Work out the finished part from the listing and answer in its coordinate system (mm). A direction names the side the tool comes from. Round coordinates to 2 decimals unless told otherwise and drop trailing zeros. Loops run counter-clockwise (first coordinate to the right, second up) from the corner with the lowest first, then second, coordinate; pieces in that order, holes last. Notation, with made-up numbers: (-29.75, -15) - (13.25, -15) arc R13 cw to (13.25, -3) - close; hole circle Ø7 at (17, 37.25). An arc over 180 degrees is marked (long way). Return JSON: item names as keys, results as strings.
from build123d import *

# Parameters (mm, degrees)
SKETCH1_R                         = 24.765
BOSS_EXTRUDE1_DEPTH               = 19.05
SKETCH2_OUTSIDE_W                 = 66.048
SKETCH2_OUTSIDE_H                 = 66.048
CUT_EXTRUDE1_DEPTH                = 9.525
F_1_4_20_TAPPED_HOLE5_D           = 5.1054
F_1_4_20_TAPPED_HOLE5_DEPTH       = 7.62
F_1_4_20_TAPPED_HOLE5_CSINK_D     = 6.731
F_1_4_20_TAPPED_HOLE5_CSINK_ANGLE = 90
F_1_4_20_TAPPED_HOLE5_TIP         = 1.533816902


with BuildPart() as part:
    # Sketch1 → Boss-Extrude1 (new body)
    with BuildSketch(Plane(origin=(0, 0, 0), x_dir=(1, 0, 0), z_dir=(0, 1, 0))):
        Circle(SKETCH1_R)
    extrude(amount=BOSS_EXTRUDE1_DEPTH)

    # Sketch2 outside → Cut-Extrude1 (cut)
    with BuildSketch(Plane(origin=(0, 19.05, 0), x_dir=(1, 0, 0), z_dir=(0, 1, 0))):
        Rectangle(SKETCH2_OUTSIDE_W, SKETCH2_OUTSIDE_H)
        with BuildLine():
            Line((-14.19414924, -18.920099441), (-9.994377531, -5.994531191))
            ThreePointArc((-9.994377531, -5.994531191), (-9.994377531, -3.247370111), (-11.609118299, -1.024870111))
            Line((-11.609118299, -1.024870111), (-22.60426338, 6.963570391))
            ThreePointArc((-22.60426338, 6.963570391), (-22.742669731, 7.389541341), (-22.380317198, 7.652805866))
            Line((-22.380317198, 7.652805866), (-8.789570457, 7.652805866))
            ThreePointArc((-8.789570457, 7.652805866), (-6.176865011, 8.501725326), (-4.562124242, 10.724225326))
            Line((-4.562124242, 10.724225326), (-0.362352533, 23.649793575))
            ThreePointArc((-0.362352533, 23.649793575), (0, 23.913058101), (0.362352533, 23.649793575))
            Line((0.362352533, 23.649793575), (4.562124242, 10.724225326))
            ThreePointArc((4.562124242, 10.724225326), (6.176865011, 8.501725326), (8.789570457, 7.652805866))
            Line((8.789570457, 7.652805866), (22.380317198, 7.652805866))
            ThreePointArc((22.380317198, 7.652805866), (22.742669731, 7.389541341), (22.60426338, 6.963570391))
            Line((22.60426338, 6.963570391), (11.609118299, -1.024870111))
            ThreePointArc((11.609118299, -1.024870111), (9.994377531, -3.247370111), (9.994377531, -5.994531191))
            Line((9.994377531, -5.994531191), (14.19414924, -18.920099441))
            ThreePointArc((14.19414924, -18.920099441), (14.055742889, -19.346070391), (13.607850526, -19.346070391))
            Line((13.607850526, -19.346070391), (2.612705446, -11.357629889))
            ThreePointArc((2.612705446, -11.357629889), (0, -10.508710429), (-2.612705446, -11.357629889))
            Line((-2.612705446, -11.357629889), (-13.607850526, -19.346070391))
            ThreePointArc((-13.607850526, -19.346070391), (-14.055742889, -19.346070391), (-14.19414924, -18.920099441))
        make_face(mode=Mode.SUBTRACT)
    extrude(amount=-CUT_EXTRUDE1_DEPTH, mode=Mode.SUBTRACT)

    # 1/4-20 Tapped Hole5
    with Locations(Plane(origin=(0, 9.525, 0), x_dir=(1, 0, 0), z_dir=(0, 1, 0))):
        with Locations((-18.117626635, -5.886773743), (-11.197309056, 15.411773743), (11.197309056, 15.411773743), (18.117626635, -5.886773743), (0, -19.05)):
            CounterSinkHole(F_1_4_20_TAPPED_HOLE5_D / 2, F_1_4_20_TAPPED_HOLE5_CSINK_D / 2, depth=F_1_4_20_TAPPED_HOLE5_DEPTH, counter_sink_angle=F_1_4_20_TAPPED_HOLE5_CSINK_ANGLE)
            with Locations((0, 0, -(F_1_4_20_TAPPED_HOLE5_DEPTH + F_1_4_20_TAPPED_HOLE5_TIP / 2))):  # 118° drill point
                Cone(0, F_1_4_20_TAPPED_HOLE5_D / 2, F_1_4_20_TAPPED_HOLE5_TIP, mode=Mode.SUBTRACT)


solid = part.part
1) Section A-A (y = 15) is taken. Give the vertices of the cut face in (x, z) (3 decimals).
Verdict:
{"outline": "(-22.604, -6.964) arc R0.381 ccw to (-22.38, -7.653) - (-8.79, -7.653) arc R4.445 cw to (-4.562, -10.724) - (-0.362, -23.65) arc R0.381 ccw to (0.362, -23.65) - (4.562, -10.724) arc R4.445 cw to (8.79, -7.653) - (22.38, -7.653) arc R0.381 ccw to (22.604, -6.964) - (11.609, 1.025) arc R4.445 cw to (9.994, 5.995) - (14.194, 18.92) arc R0.381 ccw to (13.608, 19.346) - (2.613, 11.358) arc R4.445 cw to (-2.613, 11.358) - (-13.608, 19.346) arc R0.381 ccw to (-14.194, 18.92) - (-9.994, 5.995) arc R4.445 cw to (-11.609, 1.025) - close"}
2) A tool of negligible diameter and unlimited length cuts with its end or side. For faces 4 (the cylindrical face through (-6.21, 14.35, -8.48)), 5 (the flat face through (-12.124, 14.354, 12.548)), 6 (the cylindrical face through (6.15, 14.35, -8.52)), from which of +Z, -Z, +X, -X, +Y, -Y can it reach the whole face along a straight path? Write none if from no direction.
Verdict:
{"face 4": "-Z, -X, +Y", "face 5": "-X, +Y", "face 6": "-Z, +X, +Y"}
3) Section C-C (y = 5.25) is taken. Give the vertices of the cut face in (x, z) (3 decimals), and give its area (3 significant figures).
Verdict:
{"outline": "circle Ø49.53 at (0, 0); hole circle Ø5.105 at (-18.118, 5.887); hole circle Ø5.105 at (-11.197, -15.412); hole circle Ø5.105 at (0, 19.05); hole circle Ø5.105 at (11.197, -15.412); hole circle Ø5.105 at (18.118, 5.887)", "area": "1,820 mm2"}
4) Section B-B (z = 0) is taken. Give the vertices of the cut face in (x, y) (3 decimals), and give its area (3 significant figures).
Verdict:
{"outline": "(-24.765, 0) - (24.765, 0) - (24.765, 9.525) - (13.02, 9.525) - (13.02, 19.05) - (-13.02, 19.05) - (-13.02, 9.525) - (-24.765, 9.525) - close", "area": "720 mm2"}
5) Find the intervals of material crossed by L1, parallel to Z at x = 0, y = 4.25 (3 decimals); L2, parallel to Z at x = 0, y = 11.75; L3, parallel to Y at x = 7.5, z = -13 (3 decimals), in increasing order.
Verdict:
{"L1": "z = -24.765 to 16.497, 21.603 to 24.765", "L2": "z = -23.91 to 10.51", "L3": "y = 0 to 9.525"}
6) Flat-ended cylindrical pins translate along their axes: pin 1 (3 mm diameter, centred on x = 12, y = 15, fed in from -Z); pin 2 (3 mm diameter, centred on y = 16, z = 5, fed in from +X); pin 3 (4 mm diameter, centred on y = 15, z = 2, fed in from -X). Find the tip coordinate at first contact, or state that the pin passes through.
Verdict:
{"pin 1": "stops at z = -7.65", "pin 2": "stops at x = 10.16", "pin 3": "stops at x = -13.02"}
7) Determine the mould class of faces 1 (the flat face through (0, 0, 0)), 2 (the cylindrical face through (-10.865, 5.261, -17.943)), 3 (the cylindrical face through (23.62, 4.7, -7.44)) for opening direction X: pulls with the +X half, pulls with the -X half, needs draft (parallel to the pull), parting line crosses it, or undercut.
Verdict:
{"face 1": "needs draft", "face 2": "undercut", "face 3": "parting line crosses it"}
